For this review, use the dimensioned drawing (mm, ordinates from the lowest corner) and the shaded views. A direction names the side the tool comes from. Give positions to 0.01 mm unless a question says otherwise; leave off trailing zeros. Write each loop counter-clockwise with the first axis right and the second up, starting at its lowest first coordinate (ties: lowest second). Pieces come first, ordered by that corner, then holes. Notation, with made-up numbers: M -25.5,58.5 L -7.5,58.5 A28 ccw -7.5,94.5 Z; hole C 66.5,0 d9. An arc over 180 degrees is marked long. One line per item, written item: value. Start each with the question number.
Item 1: To check wall thickness, follow probe 1 along X at (y, z) = (145, 13); probe 2 along Y at (x, z) = (5, 19.5); probe 3 along Y at (x, z) = (22.75, 16.75). State the ranges of each line that lie inside material, in increasing order.
Item 2: Consider section D-D, the plane y = 47. Write out the cut boundary in (x, z), and give its area (3 significant figures).
Item 3: Consider section B-B, the plane x = 14. Write out the cut boundary in (y, z).
Item 4: Tool access review of the marked faces 1, 2 and 3: name each direction out of +Z, -Z, +X, -X, +Y, -Y from which nothing blocks a thin tool from reaching the whole face with its end or side.
Item 5: Clearance check with flat-ended pins moving along their axes: pin 1 Ø1.5 at (y, z) = (106.5, 8.5) entering from +X; pin 2 Ø3 at (x, y) = (16, 278.5) entering from +Z; pin 3 Ø1 at (x, y) = (16.5, 158) entering from +Z. State where each tip first meets the part, or that it passes through.
Item 6: Consider section C-C, the plane y = 250. Write out the cut boundary in (x, z), and give its area (3 significant figures).
Item 7: Consider section A-A, the plane z = 14. Write out the cut boundary in (x, y).
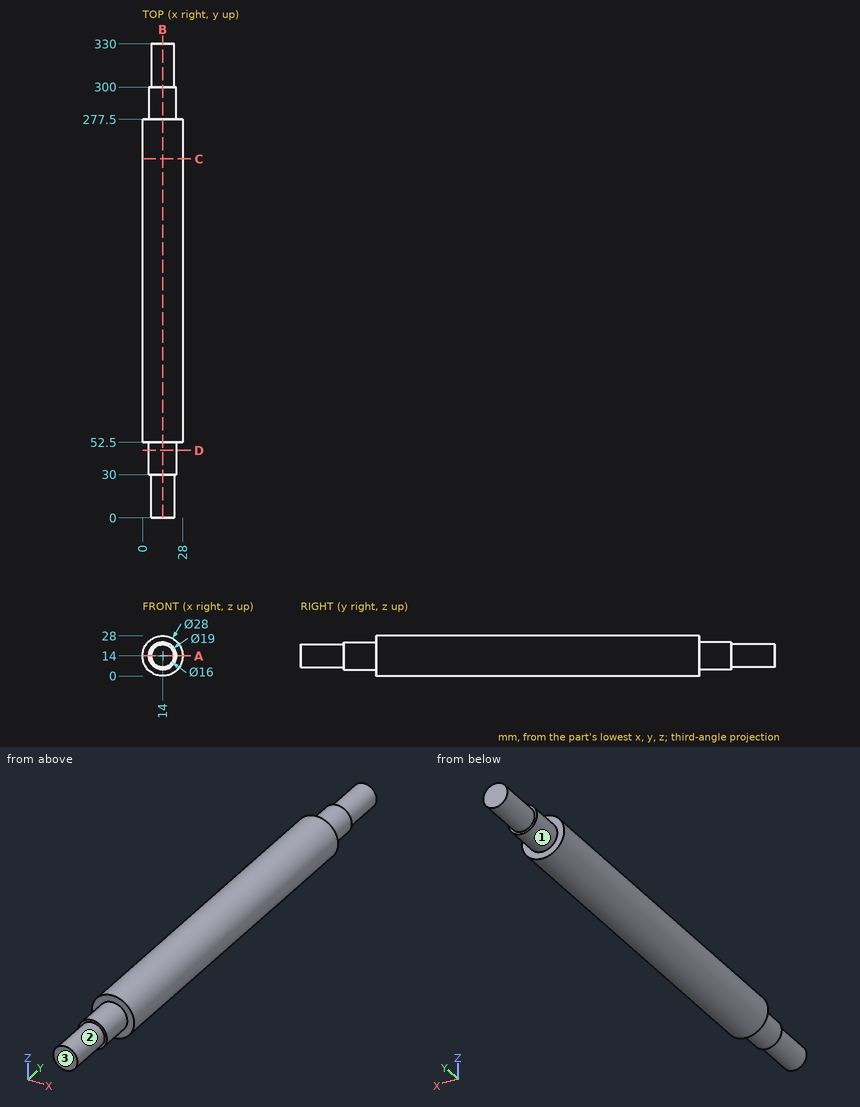
Model answer:
1. probe 1: x = 0.04 to 27.96
1. probe 2: y = 52.5 to 277.5
1. probe 3: y = 30 to 300
2. outline: C 14,14 d19
2. area: 284 mm2
3. outline: M 0,6 L 30,6 L 30,4.5 L 52.5,4.5 L 52.5,0 L 277.5,0 L 277.5,4.5 L 300,4.5 L 300,6 L 330,6 L 330,22 L 300,22 L 300,23.5 L 277.5,23.5 L 277.5,28 L 52.5,28 L 52.5,23.5 L 30,23.5 L 30,22 L 0,22 Z
4. face 1: +Y
4. face 2: -Y
4. face 3: +Z, -Z, +X, -X, -Y
5. pin 1: stops at x = 27.17
5. pin 2: stops at z = 27.97
5. pin 3: stops at z = 27.86
6. outline: C 14,14 d28
6. area: 616 mm2
7. outline: M 0,52.5 L 4.5,52.5 L 4.5,30 L 6,30 L 6,0 L 22,0 L 22,30 L 23.5,30 L 23.5,52.5 L 28,52.5 L 28,277.5 L 23.5,277.5 L 23.5,300 L 22,300 L 22,330 L 6,330 L 6,300 L 4.5,300 L 4.5,277.5 L 0,277.5 Z
